```python
from build123d import *

# Parameters (mm, degrees)
F1_DEPTH = 6.35
F3_W     = 31.75
F3_H     = 6.35
F4_DEPTH = 82.55
F6_DEPTH = 6.35


with BuildPart() as f1:
    # F0 (on Front) → F1 (new body)
    with BuildSketch(Plane.XZ):
        Polygon((-41.275, 13.647084), (-41.275, 53.975), (-111.125, 53.975), align=None)
        Polygon((0, 53.975), (-41.275, 53.975), (-41.275, 13.647084), (-41.275, -53.975), (0, -53.975), align=None)
    extrude(amount=-F1_DEPTH)

    # F2: F1 across plane


with BuildPart() as f1_1:
    add(f1.part)
    add(f1.part.mirror(Plane.YZ))

    # F3 (on Front) → F4 (join)
    with BuildSketch(Plane.XZ):
        with Locations((0, -50.8)):
            Rectangle(F3_W, F3_H)
    extrude(amount=F4_DEPTH)

    # F5 (on face) → F6 (join)
    with BuildSketch(Plane.YZ.offset(15.875)):
        Polygon((0, -22.225), (-25.4, -47.625), (0, -47.625), align=None)
    extrude(amount=-F6_DEPTH)

    # F7: F1 across plane


with BuildPart() as f1_2:
    add(f1_1.part)
    add(f1_1.part.mirror(Plane.YZ))


solid = f1_2.part
```
Geometry check sheet. Reference: the model listing, model coordinates, mm. A direction names the side the tool comes from. Round coordinates to 2 decimals unless told otherwise and drop trailing zeros. Loops run counter-clockwise (first coordinate to the right, second up) from the corner with the lowest first, then second, coordinate; pieces in that order, holes last. Notation, with made-up numbers: (59.5, -17.75) - (77.5, -17.75) arc R25 ccw to (77.5, 16.25) - close; hole circle Ø9 at (-38, -20). An arc over 180 degrees is marked (long way). Write each question's results on one line, items separated by ' | '. Start each with the question number.
Q1. Cross-section at D-D on z = -2.5. Enter the section's corners in (x, y) (3 decimals), and give its area (3 significant figures).
Q2. Cross-section at A-A on y = -21.5. Enter the section's corners in (x, z) (3 decimals), and give its area (3 significant figures).
Q3. Gauge pin test, flat ends, axial feed: P1, Ø7.5, axis at y = -12.5, z = -30, coming from the +X side (3 decimals); P2, Ø5, axis at y = 2, z = -32.5, coming from the +X side (3 decimals); P3, Ø16, axis at y = -38.5, z = -45, coming from the -X side (3 decimals). Record the tip position at first contact, or that the pin passes through.
Q4. Cross-section at C-C on x = -19. Enter the section's corners in (y, z) (3 decimals).
Q5. Cross-section at B-B on z = -39. Enter the section's corners in (x, y) (3 decimals).
Q6. Release check for a two-part mould opening along X. For faces 6 (the flat face through (15.875, -29, -50)), 7 (the flat face through (9.525, -7, -40)), 8 (the flat face through (-15.875, -29, -50)), 9 (the flat face through (-2, 3, 53.975)) record: +X half, -X half, draft (parallel to the pull), parting line (faces both ways), or undercut.
Q7. Thickness scan on line 1 (Y direction, x = -26.5, z = 16); line 2 (Z direction, x = 10, y = -39) (3 decimals); line 3 (X direction, y = -7.5, z = -49) (3 decimals). Record the ranges inside material, lowest first. Write a range as [from, to].
Q8. Access from +Z, -Z, +X, -X, +Y, -Y to the whole of each face (thin tool, end or side, straight path). Record for faces 1 (the flat face through (1, -29, -53.975)), 2 (the flat face through (-9.525, -7, -40)), 3 (the flat face through (41.275, 3, -20)), 4 (the flat face through (-41.275, 3, -20)), 5 (the flat face through (2, 6.35, 13)).
Answers below:
1) outline: (-41.275, 0) - (41.275, 0) - (41.275, 6.35) - (-41.275, 6.35) - close | area: 524 mm²
2) outline: (-15.875, -53.975) - (15.875, -53.975) - (15.875, -43.725) - (9.525, -43.725) - (9.525, -47.625) - (-9.525, -47.625) - (-9.525, -43.725) - (-15.875, -43.725) - close | area: 251 mm²
3) P1: stops at x = 15.875 | P2: stops at x = 41.275 | P3: stops at x = -15.875
4) outline: (0, -53.975) - (6.35, -53.975) - (6.35, 53.975) - (0, 53.975) - close
5) outline: (-41.275, 0) - (-15.875, 0) - (-15.875, -16.775) - (-9.525, -16.775) - (-9.525, 0) - (9.525, 0) - (9.525, -16.775) - (15.875, -16.775) - (15.875, 0) - (41.275, 0) - (41.275, 6.35) - (-41.275, 6.35) - close
6) face 6: +X half | face 7: undercut | face 8: -X half | face 9: draft
7) line 1: y = [0, 6.35] | line 2: z = [-53.975, -47.625] | line 3: x = [-15.875, 15.875]
8) face 1: -Z, +X, -X, +Y, -Y | face 2: +Z, -Y | face 3: -Z, +X, +Y, -Y | face 4: -Z, -X, +Y, -Y | face 5: +Z, -Z, +X, -X, +Y
